Verification items for the finished model (mm, model axes). A direction names the side the tool comes from. Round coordinates to 2 decimals unless told otherwise and drop trailing zeros. Order: outer loops, then holes, each group sorted by start corner. A loop starts at its lowest first (then second) coordinate and runs counter-clockwise, first axis right, second up. Notation, with made-up numbers: (34.25, 55.5) -> (59.25, 55.5) arc R18 cw to (59.25, 80.5) -> close; hole circle Ø9 at (1, 84). An arc over 180 degrees is marked (long way). Put each result on its own line as item: value.
```python
from build123d import *

# Parameters (mm, degrees)
ESQUISSE1_R             = 25
BOSS_EXTRU_1_DEPTH      = 19.1
ESQUISSE2_R             = 18.3
BOSS_EXTRU_2_DEPTH      = 0.5
CONG_1_R                = 1.5
ESQUISSE3_R             = 18.3
BOSS_EXTRU_3_DEPTH      = 0.5
ESQUISSE4_R             = 17.5
ENL_V_MAT_EXTRU_1_DEPTH = 7.45
ESQUISSE5_R             = 17.5
ENL_V_MAT_EXTRU_2_DEPTH = 7.45
ESQUISSE6_R             = 7.5
BOSS_EXTRU_4_DEPTH      = 8.9
BOSS_EXTRU_4_TAPER      = 6
CONG_2_R                = 1.5
ESQUISSE7_R             = 7.5
BOSS_EXTRU_5_DEPTH      = 8.9
BOSS_EXTRU_5_TAPER      = 6
CONG_3_R                = 1.5
ESQUISSE8_R             = 3
ENL_V_MAT_EXTRU_3_DEPTH = 28.9


with BuildPart() as part:
    # Esquisse1 → Boss.-Extru.1 (new body)
    with BuildSketch(Plane(origin=(0, 0, 0), x_dir=(0, 0, -1), z_dir=(1, 0, 0))):
        Circle(ESQUISSE1_R)
    extrude(amount=BOSS_EXTRU_1_DEPTH)

    # Esquisse2 → Boss.-Extru.2 (add)
    with BuildSketch(Plane(origin=(19.1, 0, 0), x_dir=(0, 0, -1), z_dir=(1, 0, 0))):
        Circle(ESQUISSE2_R)
    extrude(amount=BOSS_EXTRU_2_DEPTH)

    # Congé1
    cong_1_edges = [part.edges().sort_by_distance(p)[0] for p in [
        (0, 0, 25),
        (19.1, 0, 25),
    ]]
    fillet(cong_1_edges, radius=CONG_1_R)

    # Esquisse3 → Boss.-Extru.3 (add)
    with BuildSketch(Plane.ZY):
        Circle(ESQUISSE3_R)
    extrude(amount=BOSS_EXTRU_3_DEPTH)

    # Esquisse4 → Enlèv. mat.-Extru.1 (cut)
    with BuildSketch(Plane.ZY.offset(0.5)):
        Circle(ESQUISSE4_R)
    extrude(amount=-ENL_V_MAT_EXTRU_1_DEPTH, mode=Mode.SUBTRACT)

    # Esquisse5 → Enlèv. mat.-Extru.2 (cut)
    with BuildSketch(Plane(origin=(19.6, 0, 0), x_dir=(0, 0, -1), z_dir=(1, 0, 0))):
        Circle(ESQUISSE5_R)
    extrude(amount=-ENL_V_MAT_EXTRU_2_DEPTH, mode=Mode.SUBTRACT)

    # Esquisse6 → Boss.-Extru.4 (add)
    with BuildSketch(Plane(origin=(12.15, 0, 0), x_dir=(0, 0, -1), z_dir=(1, 0, 0))):
        Circle(ESQUISSE6_R)
    extrude(amount=BOSS_EXTRU_4_DEPTH, taper=BOSS_EXTRU_4_TAPER)

    # Congé2
    cong_2_edges = [part.edges().sort_by_distance(p)[0] for p in [
        (12.15, 0, 7.5),
    ]]
    fillet(cong_2_edges, radius=CONG_2_R)

    # Esquisse7 → Boss.-Extru.5 (add)
    with BuildSketch(Plane.ZY.offset(-6.95)):
        Circle(ESQUISSE7_R)
    extrude(amount=BOSS_EXTRU_5_DEPTH, taper=BOSS_EXTRU_5_TAPER)

    # Congé3
    cong_3_edges = [part.edges().sort_by_distance(p)[0] for p in [
        (6.95, 0, -7.5),
    ]]
    fillet(cong_3_edges, radius=CONG_3_R)

    # Esquisse8 → Enlèv. mat.-Extru.3 (cut)
    with BuildSketch(Plane.ZY.offset(1.95)):
        Circle(ESQUISSE8_R)
    extrude(amount=-ENL_V_MAT_EXTRU_3_DEPTH, mode=Mode.SUBTRACT)


solid = part.part
```
Item 1: Release check for a two-part mould opening along Y. For faces 4 (the face through (19.35, 15.43, -9.84)), 5 (the face through (15.927, -10.648, 13.887)), 6 (the face through (19.6, -1, -18)), 7 (the face through (0.94, -4.18, -5.45)) record: pulls with the +Y half, pulls with the -Y half, needs draft (parallel to the pull), parting line crosses it, or undercut.
Geometry check:
face 4: parting line crosses it
face 5: undercut
face 6: needs draft
face 7: undercut
Item 2: Sectioned sample at A-A, the plane x = 0.75. Record the boundary of the cut face in (y, z).
Geometry check:
outline: circle Ø49.6 at (0, 0); circle Ø13.7 at (0, 0); hole circle Ø35 at (0, 0); hole circle Ø6 at (0, 0)
Item 3: Tool access check on faces 1 (the face through (12.15, 4.13, 8.02)), 2 (the face through (-0.5, -1, 18)), 3 (the face through (-1.95, -1, 3)). Record the directions out of +Z, -Z, +X, -X, +Y, -Y that give a thin tool (end or side, any length) a straight path to the whole face; none if there is none.
Geometry check:
face 1: +X
face 2: -X
face 3: +Z, -Z, -X, +Y, -Y
Item 4: Material ranges on line 1 along Y through (x, z) = (13, 0); line 2 along Y through (x, z) = (17.5, 2.5); line 3 along Z through (x, y) = (6, 6), recorded low to high.
Geometry check:
line 1: -25 to -17.5, -7.5 to -3, 3 to 7.5, 17.5 to 25
line 2: -24.87 to -17.32, -6.47 to -1.66, 1.66 to 6.47, 17.32 to 24.87
line 3: -24.27 to -16.44, -4.42 to 4.42, 16.44 to 24.27
Item 5: Depth check by flat-ended pin: pin 1 Ø4 at (x, y) = (12.5, 18) entering from -Z; pin 2 Ø6 at (x, z) = (9.5, 5.5) entering from -Y; pin 3 Ø6 at (x, z) = (15, -7.5) entering from +Y. Enter the tip coordinate at first touch or a pass-through.
Geometry check:
pin 1: z = -19.21
pin 2: y = -24.87
pin 3: y = 24.59
Item 6: Sectioned sample at C-C, the plane x = 5. Record the boundary of the cut face in (y, z), then the cut area to 3 significant figures.
Geometry check:
outline: circle Ø50 at (0, 0); circle Ø14.59 at (0, 0); hole circle Ø35 at (0, 0); hole circle Ø6 at (0, 0)
area: 1,140 mm2
Item 7: Sectioned sample at B-B, the plane x = 8. Record the boundary of the cut face in (y, z).
Geometry check:
outline: circle Ø50 at (0, 0); hole circle Ø6 at (0, 0)
